from build123d import *

# Parameters (mm, degrees)
F1_DEPTH = 10
F3_D     = 3.3
F5_D     = 3.3
F6_DEPTH = 4


with BuildPart() as f1:
    # F0 (on Front) → F1 (new body, symmetric)
    with BuildSketch(Plane.XZ):
        Polygon((10.5, 0.9), (10.5, 2.5), (-10.5, 2.5), (-10.5, 0.9), (-10.5, -0.9), (-10.5, -2.5), (10.5, -2.5), (10.5, -0.9), align=None)
        with BuildLine():
            ThreePointArc((10.5, -0.9), (11.4, 0), (10.5, 0.9))
            Line((10.5, 0.9), (10.5, -0.9))
        make_face()
        with BuildLine():
            Line((-10.5, -0.9), (-10.5, 0.9))
            ThreePointArc((-10.5, 0.9), (-11.4, 0), (-10.5, -0.9))
        make_face()
    extrude(amount=F1_DEPTH, both=True)

    # F3 (through all)
    with Locations(Plane.XY.offset(2.5)):
        with Locations((0, 0)):
            Hole(F3_D / 2)

    # F5 (through all)
    with Locations(Plane.XZ.offset(10)):
        with Locations((-6.5, 0), (6.5, 0)):
            Hole(F5_D / 2)

    # F4 (on face) → F6 (cut)
    with BuildSketch(Plane.XZ.offset(10)):
        Polygon((-3.45, 0), (-4.975, 2.6413774815), (-8.025, 2.6413774815), (-9.55, 0), (-8.025, -2.6413774815), (-4.975, -2.6413774815), align=None)
        Polygon((4.975, 2.6413774815), (3.45, 0), (4.975, -2.6413774815), (8.025, -2.6413774815), (9.55, 0), (8.025, 2.6413774815), align=None)
    extrude(amount=-F6_DEPTH, mode=Mode.SUBTRACT)


solid = f1.part
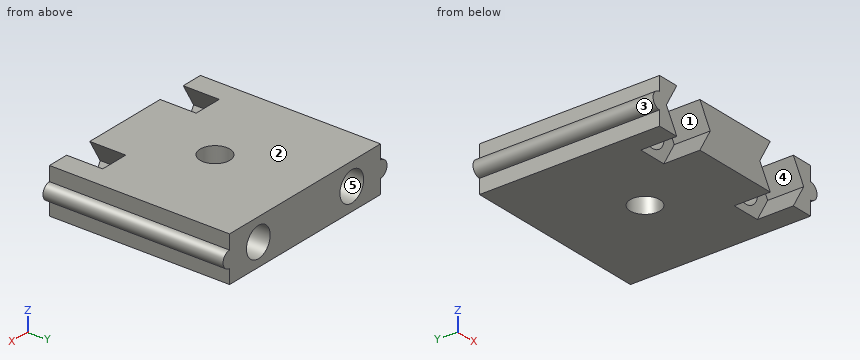
Here's how the part is built. I have some questions about the finished solid (model axes, mm). Face numbers are marked on the shaded views. A direction names the side the tool comes from. Round coordinates to 2 decimals unless told otherwise and drop trailing zeros. Order: outer loops, then holes, each group sorted by start corner. A loop starts at its lowest first (then second) coordinate and runs counter-clockwise, first axis right, second up. Notation, with made-up numbers: M -32,-35 L 8,-35 A29 cw 8,-9 Z; hole C -16.5,34 d11. An arc over 180 degrees is marked long. Return JSON: item names as keys, results as strings. Group by question number.
1. If we section it at D-D on y = -7: List the corners of the cut face in (x, z) for me, then the cut area to 3 significant figures.
2. I'm going to push flat-ended pins straight in: pin 1 Ø1 at (y, z) = (6, 1) entering from -X; pin 2 Ø0.5 at (y, z) = (-4.5, 1.5) entering from +X; pin 3 Ø1.5 at (x, z) = (5, -1) entering from -Y. Where does each tip first touch, or does it pass through?
3. Please list where these lines run through material, in increasing order: probe 1 along X at (y, z) = (-1, -1); probe 2 along X at (y, z) = (1, -0.7); probe 3 along Z at (x, y) = (-6.5, 3).
4. If we section it at B-B on x = 6.5: List the corners of the cut face in (y, z) for me, then the cut area to 3 significant figures.
5. On a 3-axis mill with a long thin cutter (end or side, diameter ignored), from which of +Z, -Z, +X, -X, +Y, -Y can I reach the whole of each face in a straight line? I mean the marked faces 4 and 5. Say none if no direction works.
6. If we section it at C-C on z = 1.15: List the corners of the cut face in (x, y) for me, then the cut area to 3 significant figures.
7. If we section it at A-A on y = 0: List the corners of the cut face in (x, z) for me, then the cut area to 3 significant figures.
8. If we mould it in two halves opening along X, with no side actions, what happens to the marked faces 1, 2 and 3? For each: pulls with the +X half, pulls with the -X half, needs draft (parallel to the pull), parting line crosses it, or undercut.
Reply:
{
 "1": {"outline": "M -10.5,-2.5 L -8.11,-2.5 L -9.55,0 L -8.11,2.5 L -10.5,2.5 L -10.5,0.9 A0.9 ccw -10.5,-0.9 Z; M -4.89,-2.5 L 4.89,-2.5 L 3.45,0 L 4.89,2.5 L -4.89,2.5 L -3.45,0 Z; M 8.11,-2.5 L 10.5,-2.5 L 10.5,-0.9 A0.9 ccw 10.5,0.9 L 10.5,2.5 L 8.11,2.5 L 9.55,0 Z", "area": "61.0 mm^2"},
 "2": {"pin 1": "x = -11.25", "pin 2": "x = 10.5", "pin 3": "y = -6"},
 "3": {"probe 1": "-10.5 to -7.81, -5.19 to -1.31, 1.31 to 5.19, 7.81 to 10.5", "probe 2": "-11.07 to -7.99, -5.01 to -1.31, 1.31 to 5.01, 7.99 to 11.07", "probe 3": "-2.5 to -1.65, 1.65 to 2.5"},
 "4": {"outline": "M -6,-2.5 L 10,-2.5 L 10,-1.65 L -6,-1.65 Z; M -6,1.65 L 10,1.65 L 10,2.5 L -6,2.5 Z", "area": "27.2 mm^2"},
 "5": {"face 4": "-Y", "face 5": "+Y, -Y"},
 "6": {"outline": "M -10.5,-10 L -8.89,-10 L -8.89,-6 L -7.68,-6 L -7.68,10 L -10.5,10 Z; M -5.32,-6 L -4.11,-6 L -4.11,-10 L 4.11,-10 L 4.11,-6 L 5.32,-6 L 5.32,10 L -5.32,10 Z; M 7.68,-6 L 8.89,-6 L 8.89,-10 L 10.5,-10 L 10.5,10 L 7.68,10 Z; hole C 0,0 d3.3", "area": "298 mm^2"},
 "7": {"outline": "M -10.5,-2.5 L -1.65,-2.5 L -1.65,2.5 L -10.5,2.5 L -10.5,0.9 A0.9 ccw -10.5,-0.9 Z; M 1.65,-2.5 L 10.5,-2.5 L 10.5,-0.9 A0.9 ccw 10.5,0.9 L 10.5,2.5 L 1.65,2.5 Z; hole C -6.5,0 d3.3; hole C 6.5,0 d3.3", "area": "73.9 mm^2"},
 "8": {"face 1": "undercut", "face 2": "needs draft", "face 3": "pulls with the -X half"}
}
